from build123d import *

# Parameters (mm, degrees)
SKETCH1_R           = 5
BOSS_EXTRUDE1_DEPTH = 80
SCALE1_SCALE        = 1.9329
BOSS_EXTRUDE2_START = 0.6
SKETCH3_R           = 25.1277
BOSS_EXTRUDE2_DEPTH = 0.6
SCALE2_SCALE        = 1.5


with BuildPart() as part:
    # Sketch1 → Boss-Extrude1 (new body)
    with BuildSketch(Plane.XY):
        Circle(SKETCH1_R)
    extrude(amount=BOSS_EXTRUDE1_DEPTH)

    # Sketch2 → Revolve1 (revolve)
    with BuildSketch(Plane(origin=(0, 0, 0), x_dir=(1, 0, 0), z_dir=(0, 1, 0))):
        Polygon((0, -66), (0, -68), (-5, -68), (-13, -68), (-13, -66), align=None)
    revolve(axis=Axis((0, 0, 66), (0, 0, 1)))


with BuildPart() as part_1:
    # Scale1: scaled about (0, 0, 43.398601399)
    add(part.part.scale(SCALE1_SCALE).moved(Location((0, 0, -40.486555245))))

    # Sketch3 → Boss-Extrude2 (add)
    with BuildSketch(Plane(origin=(0, 0, 87.084844755), x_dir=(-1, 0, 0), z_dir=(0, 0, -1)).offset(BOSS_EXTRUDE2_START)):
        Circle(SKETCH3_R)
    extrude(amount=-BOSS_EXTRUDE2_DEPTH)

    # Sketch4 → Cut-Revolve1 (revolve, cut)
    with BuildSketch(Plane(origin=(0, 0, 0), x_dir=(0, 0, -1), z_dir=(1, 0, 0)), mode=Mode.PRIVATE) as cut_revolve1_sk:
        Polygon((-76.705174755, 26.6900619), (-76.705174755, 0), (46.736883237, 0), (46.736883237, 27.883866585), align=None)
    revolve(cut_revolve1_sk.sketch.rotate(Axis((0, 0, 76.705174755), (0, 0, -1)), 270), axis=Axis((0, 0, 76.705174755), (0, 0, -1)), mode=Mode.SUBTRACT)


with BuildPart() as part_2:
    # Scale2: scaled about (0, 0, 92.693679073)
    add(part_1.part.scale(SCALE2_SCALE).moved(Location((0, 0, -46.346839536))))


solid = part_2.part
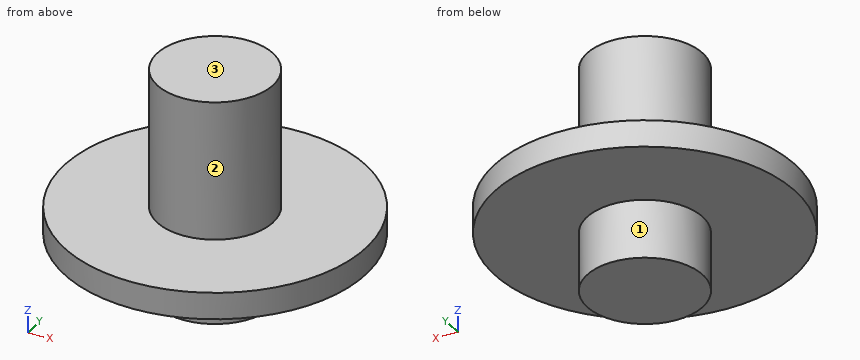
Could you check a few things on this model? Use its own coordinates, in mm. Face numbers are marked on the shaded views. A direction names the side the tool comes from. Give positions to 0.01 mm unless a question says otherwise; leave off trailing zeros. Order: outer loops, then holes, each group sorted by start corner. A loop starts at its lowest first (then second) coordinate and runs counter-clockwise, first axis right, second up.
1. I need wall thicknesses on L1, parallel to X at y = -0.5, z = 112.5; L2, parallel to Z at x = -32, y = 10; L3, parallel to X at y = -3.5, z = 89. Which ranges of each line are inside material? Lowest first, please.
Answers below:
L1: x = -14.49 to 14.49
L2: z = 83.38 to 90.08
L3: x = -37.53 to 37.53
2. For pin 1 (10 mm diameter, centred on x = 10, z = 97.5, fed in from +Y); pin 2 (1 mm diameter, centred on x = 8, y = -14, fed in from +Z); pin 3 (2 mm diameter, centred on y = 0, z = 80.5, fed in from -X), each with a flat end and sliding along its axis, tell me the tip position at first contact or that it passes through.
Answers below:
pin 1: stops at y = 13.61
pin 2: stops at z = 90.08
pin 3: stops at x = -14.5
3. Suppose I cut it at D-D (z = 80.5). Write out the boundary of the cut face in (x, y).
Answers below:
outline: circle Ø28.99 at (0, 0)
4. Suppose I cut it at C-C (z = 89). Write out the boundary of the cut face in (x, y), plus the area to 3 significant figures.
Answers below:
outline: circle Ø75.38 at (0, 0)
area: 4,460 mm2
5. Suppose I cut it at A-A (y = 0). Write out the boundary of the cut face in (x, z), plus the area to 3 significant figures.
Answers below:
outline: (-37.69, 83.38) - (-14.5, 83.38) - (-14.5, 68.71) - (14.5, 68.71) - (14.5, 83.38) - (37.69, 83.38) - (37.69, 90.08) - (14.5, 90.08) - (14.5, 124.87) - (-14.5, 124.87) - (-14.5, 90.08) - (-37.69, 90.08) - close
area: 1,940 mm2
6. Which directions (+Z, -Z, +X, -X, +Y, -Y) give clear straight access to the entire face, cutting with the end or side of a thin tool? Please do the marked faces 1, 2 and 3.
Answers below:
face 1: -Z
face 2: +Z
face 3: +Z, +X, -X, +Y, -Y
